```python
from build123d import *

# Parameters (mm, degrees)
SKETCH2_R           = 1.5
SKETCH2_R_2         = 32.25
BOSS_EXTRUDE1_DEPTH = 2
SKETCH3_R           = 45
CUT_EXTRUDE1_DEPTH  = 74.566296631


with BuildPart() as part:
    # Sketch2 → Boss-Extrude1 (new body)
    with BuildSketch(Plane(origin=(0, 0, 0), x_dir=(1, 0, 0), z_dir=(0, 1, 0))):
        with BuildLine():
            Line((17.897079586, 48.929734976), (40.149284407, 43.651218265))
            ThreePointArc((40.149284407, 43.651218265), (42.540265174, 42.312242187), (43.866371506, 39.91409958))
            Line((43.866371506, 39.91409958), (49.02521675, 17.633846579))
            ThreePointArc((49.02521675, 17.633846579), (49.23478351, 16.809026698), (49.479249782, 15.993868858))
            ThreePointArc((49.479249782, 15.993868858), (51.999812242, -0.139738387), (49.392575566, -16.259565766))
            ThreePointArc((49.392575566, -16.259565766), (49.143731732, -17.073397941), (48.929734976, -17.897079586))
            Line((48.929734976, -17.897079586), (43.651218265, -40.149284407))
            ThreePointArc((43.651218265, -40.149284407), (42.312242187, -42.540265174), (39.91409958, -43.866371506))
            Line((39.91409958, -43.866371506), (17.633846579, -49.02521675))
            ThreePointArc((17.633846579, -49.02521675), (16.809026698, -49.23478351), (15.993868858, -49.479249782))
            ThreePointArc((15.993868858, -49.479249782), (-0.139738387, -51.999812242), (-16.259565766, -49.392575566))
            ThreePointArc((-16.259565766, -49.392575566), (-17.073397941, -49.143731732), (-17.897079586, -48.929734976))
            Line((-17.897079586, -48.929734976), (-40.149284407, -43.651218265))
            ThreePointArc((-40.149284407, -43.651218265), (-42.540265174, -42.312242187), (-43.866371506, -39.91409958))
            Line((-43.866371506, -39.91409958), (-49.02521675, -17.633846579))
            ThreePointArc((-49.02521675, -17.633846579), (-49.23478351, -16.809026698), (-49.479249782, -15.993868858))
            ThreePointArc((-49.479249782, -15.993868858), (-51.999812242, 0.139738387), (-49.392575566, 16.259565766))
            ThreePointArc((-49.392575566, 16.259565766), (-49.143731732, 17.073397941), (-48.929734976, 17.897079586))
            Line((-48.929734976, 17.897079586), (-43.651218265, 40.149284407))
            ThreePointArc((-43.651218265, 40.149284407), (-42.312242187, 42.540265174), (-39.91409958, 43.866371506))
            Line((-39.91409958, 43.866371506), (-17.633846579, 49.02521675))
            ThreePointArc((-17.633846579, 49.02521675), (-16.809026698, 49.23478351), (-15.993868858, 49.479249782))
            ThreePointArc((-15.993868858, 49.479249782), (-8.026622704, 51.3767781), (0.139738387, 51.999812242))
            ThreePointArc((0.139738387, 51.999812242), (8.302633013, 51.332896714), (16.259565766, 49.392575566))
            ThreePointArc((16.259565766, 49.392575566), (17.073397941, 49.143731732), (17.897079586, 48.929734976))
        make_face()
        with Locations(Location((-38.8907, 38.8907, 0), (0, 0, 270))):
            Circle(SKETCH2_R, mode=Mode.SUBTRACT)
        with Locations(Location((38.8907, 38.8907, 0), (0, 0, 90))):
            Circle(SKETCH2_R, mode=Mode.SUBTRACT)
        with Locations(Location((38.8907, -38.8907, 0), (0, 0, 270))):
            Circle(SKETCH2_R, mode=Mode.SUBTRACT)
        with Locations(Location((-38.8907, -38.8907, 0), (0, 0, 90))):
            Circle(SKETCH2_R, mode=Mode.SUBTRACT)
        with Locations(Location((-33.323403491, 9.101105168, 0), (0, 0, 270))):
            Circle(SKETCH2_R, mode=Mode.SUBTRACT)
        with Locations(Location((24.543490023, 24.30836138, 0), (0, 0, 270))):
            Circle(SKETCH2_R, mode=Mode.SUBTRACT)
        with Locations(Location((8.779913467, -33.409466548, 0), (0, 0, 270))):
            Circle(SKETCH2_R, mode=Mode.SUBTRACT)
        with Locations(Location((0, 0, 0), (0, 0, 270))):
            Circle(SKETCH2_R_2, mode=Mode.SUBTRACT)
        with Locations(Location((0, 38.8907, 0), (0, 0, 270))):
            Circle(SKETCH2_R, mode=Mode.SUBTRACT)
        with Locations(Location((38.8907, 0, 0), (0, 0, 270))):
            Circle(SKETCH2_R, mode=Mode.SUBTRACT)
        with Locations(Location((0, -38.8907, 0), (0, 0, 270))):
            Circle(SKETCH2_R, mode=Mode.SUBTRACT)
        with Locations(Location((-38.8907, 0, 0), (0, 0, 270))):
            Circle(SKETCH2_R, mode=Mode.SUBTRACT)
    extrude(amount=BOSS_EXTRUDE1_DEPTH)

    # Sketch3 → Cut-Extrude1 (cut, through all)
    with BuildSketch(Plane(origin=(0, 2, 0), x_dir=(1, 0, 0), z_dir=(0, 1, 0))):
        with BuildLine():
            Line((-43.651218265, 40.149284407), (-48.929734976, 17.897079586))
            ThreePointArc((-48.929734976, 17.897079586), (-49.143731732, 17.073397941), (-49.392575566, 16.259565766))
            ThreePointArc((-49.392575566, 16.259565766), (-51.999812242, 0.139738387), (-49.479249782, -15.993868858))
            ThreePointArc((-49.479249782, -15.993868858), (-49.23478351, -16.809026698), (-49.02521675, -17.633846579))
            Line((-49.02521675, -17.633846579), (-43.866371506, -39.91409958))
            ThreePointArc((-43.866371506, -39.91409958), (-42.540265174, -42.312242187), (-40.149284407, -43.651218265))
            Line((-40.149284407, -43.651218265), (-17.897079586, -48.929734976))
            ThreePointArc((-17.897079586, -48.929734976), (-17.073397941, -49.143731732), (-16.259565766, -49.392575566))
            ThreePointArc((-16.259565766, -49.392575566), (-0.139738387, -51.999812242), (15.993868858, -49.479249782))
            ThreePointArc((15.993868858, -49.479249782), (16.809026698, -49.23478351), (17.633846579, -49.02521675))
            Line((17.633846579, -49.02521675), (39.91409958, -43.866371506))
            ThreePointArc((39.91409958, -43.866371506), (42.312242187, -42.540265174), (43.651218265, -40.149284407))
            Line((43.651218265, -40.149284407), (48.929734976, -17.897079586))
            ThreePointArc((48.929734976, -17.897079586), (49.143731732, -17.073397941), (49.392575566, -16.259565766))
            ThreePointArc((49.392575566, -16.259565766), (51.999812242, -0.139738387), (49.479249782, 15.993868858))
            ThreePointArc((49.479249782, 15.993868858), (49.23478351, 16.809026698), (49.02521675, 17.633846579))
            Line((49.02521675, 17.633846579), (43.866371506, 39.91409958))
            ThreePointArc((43.866371506, 39.91409958), (42.540265174, 42.312242187), (40.149284407, 43.651218265))
            Line((40.149284407, 43.651218265), (17.897079586, 48.929734976))
            ThreePointArc((17.897079586, 48.929734976), (17.073397941, 49.143731732), (16.259565766, 49.392575566))
            ThreePointArc((16.259565766, 49.392575566), (0.139738387, 51.999812242), (-15.993868858, 49.479249782))
            ThreePointArc((-15.993868858, 49.479249782), (-16.809026698, 49.23478351), (-17.633846579, 49.02521675))
            Line((-17.633846579, 49.02521675), (-39.91409958, 43.866371506))
            ThreePointArc((-39.91409958, 43.866371506), (-42.312242187, 42.540265174), (-43.651218265, 40.149284407))
        make_face()
        with Locations(Location((0, 0, 0), (0, 0, 270))):
            Circle(SKETCH3_R, mode=Mode.SUBTRACT)
    extrude(amount=-CUT_EXTRUDE1_DEPTH, mode=Mode.SUBTRACT)


solid = part.part
```
Geometry check sheet. Reference: the model listing, model coordinates, mm. Coordinates: 2 decimals unless noted, no trailing zeros. Order: outer loops, then holes, each group sorted by start corner. A loop starts at its lowest first (then second) coordinate and runs counter-clockwise, first axis right, second up. Notation, with made-up numbers: (-6.5, 78) - (25.5, 78) arc R18 cw to (25.5, 89) - close; hole circle Ø8 at (-25, -24.5). An arc over 180 degrees is marked (long way). Answer in a Markdown table with one row per item. Add a question column.
1. Material ranges on L1, parallel to Z at x = 9.5, y = 1.35; L2, parallel to X at y = 1.7, z = -12.5; L3, parallel to X at y = 0.65, z = 20.5, recorded low to high. Write a range as [from, to].
2. Section check C-C (y = 1.2). Give the number of separate pieces and of enclosed holes in the cut face, plus the area to 3 significant figures.
3. Section check B-B (x = 0). Enter the section's corners in (y, z).
4. Gauge pin test, flat ends, axial feed: pin 1 Ø12 at (x, z) = (-4.5, 31) entering from -Y; pin 2 Ø2.5 at (x, z) = (-38.89, 0) entering from -Y; pin 3 Ø1 at (x, y) = (20, 1) entering from +Z. Record the tip position at first contact, or that the pin passes through.
5. Section check A-A (z = 0). Enter the section's corners in (x, y).
6. Draft check along Z on faces 1 (the face through (26.03, 0.99, -24.5)), 2 (the face through (-17.235, 1.014, 41.569)), 3 (the face through (-13, 2, -30)). Enter one of: +Z half, -Z half, draft (parallel to the pull), parting line (faces both ways), or undercut.
7. Section check D-D (z = -15.5). Enter the section's corners in (x, y).
Data:
| question | item | result |
|---|---|---|
| 1 | L1 | z = [-43.99, -30.82], [30.82, 32.09], [34.73, 43.99] |
| 1 | L2 | x = [-43.23, -29.73], [29.73, 43.23] |
| 1 | L3 | x = [-40.06, -24.9], [24.9, 40.06] |
| 2 | separate pieces | 1 |
| 2 | enclosed holes | 8 |
| 2 | area | 3,040 mm² |
| 3 | outline | (0, -45) - (2, -45) - (2, -40.39) - (0, -40.39) - close; (0, -37.39) - (2, -37.39) - (2, -32.25) - (0, -32.25) - close; (0, 32.25) - (2, 32.25) - (2, 37.39) - (0, 37.39) - close; (0, 40.39) - (2, 40.39) - (2, 45) - (0, 45) - close |
| 4 | pin 1 | stops at y = 0 |
| 4 | pin 2 | passes through |
| 4 | pin 3 | stops at z = 40.56 |
| 5 | outline | (-45, 0) - (-40.39, 0) - (-40.39, 2) - (-45, 2) - close; (-37.39, 0) - (-32.25, 0) - (-32.25, 2) - (-37.39, 2) - close; (32.25, 0) - (37.39, 0) - (37.39, 2) - (32.25, 2) - close; (40.39, 0) - (45, 0) - (45, 2) - (40.39, 2) - close |
| 6 | face 1 | undercut |
| 6 | face 2 | parting line |
| 6 | face 3 | draft |
| 7 | outline | (-42.25, 0) - (-28.28, 0) - (-28.28, 2) - (-42.25, 2) - close; (28.28, 0) - (42.25, 0) - (42.25, 2) - (28.28, 2) - close |
